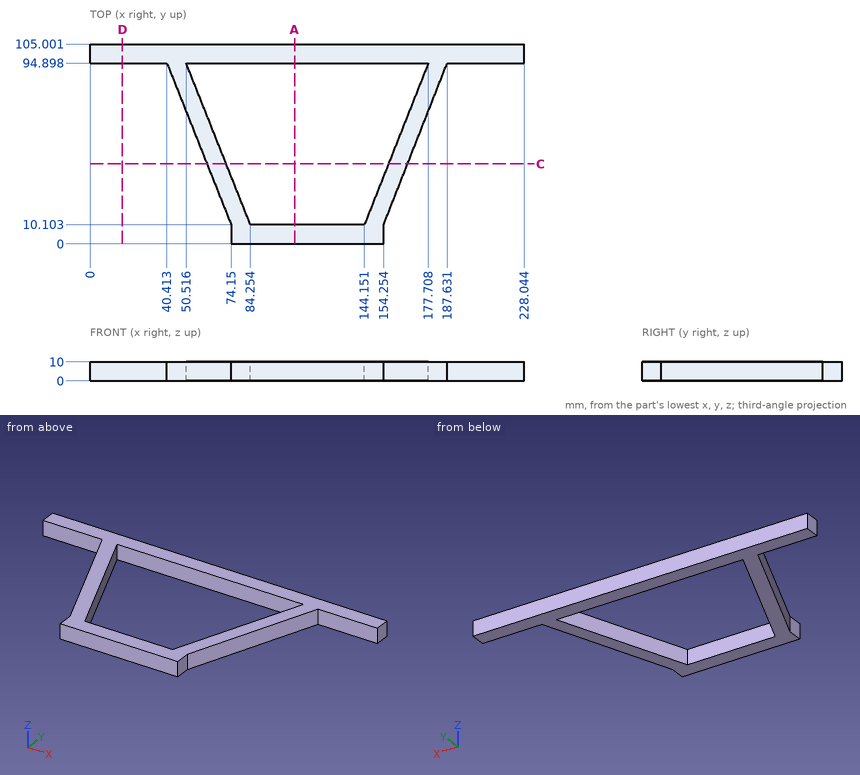
Study the drawing (mm; zero at the part's minimum x, y, z) and answer. Round coordinates to 2 decimals unless told otherwise and drop trailing zeros. Write each loop counter-clockwise with the first axis right and the second up, starting at its lowest first coordinate (ties: lowest second). Pieces come first, ordered by that corner, then holes.
Q1. Flat-ended cylindrical pins translate along their axes: P1, Ø3, axis at x = 12.5, z = 3.5, coming from the -Y side; P2, Ø5, axis at y = 49, z = 2, coming from the +X side; P3, Ø3, axis at y = 3, z = 3, coming from the +X side. Find the tip coordinate at first contact, or state that the pin passes through.
Values:
P1: stops at y = 94.9
P2: stops at x = 170.55
P3: stops at x = 154.25
Q2. Find section C-C on y = 42. Determine the outline of the cut face in (x, z) (1 decimal), and give its area (3 significant figures).
Values:
outline: (61.5, 0) - (71.6, 0) - (71.6, 10) - (61.5, 10) - close; (156.8, 0) - (166.8, 0) - (166.8, 10) - (156.8, 10) - close
area: 201 mm2
Q3. Find section A-A on x = 107.5. Determine the outline of the cut face in (y, z), and give its area (3 significant figures).
Values:
outline: (0, 0) - (10.1, 0) - (10.1, 10) - (0, 10) - close; (94.9, 0) - (105, 0) - (105, 10) - (94.9, 10) - close
area: 202 mm2
Q4. Straight lines are drawn through the part: line 1 (Y direction, x = 102, z = 6.75); line 2 (X direction, y = 27.5, z = 6) (1 decimal); line 3 (X direction, y = 33, z = 7.5) (1 decimal). For each, find the intervals that lie inside material, in ascending order.
Values:
line 1: y = 0 to 10.1, 94.9 to 105
line 2: x = 67.2 to 77.3, 151 to 161.1
line 3: x = 65 to 75.1, 153.2 to 163.3
Q5. Find section D-D on x = 17. Determine the outline of the cut face in (y, z).
Values:
outline: (94.9, 0) - (105, 0) - (105, 10) - (94.9, 10) - close
